Check sheet for the modelled part. Datum: model origin and axes. Units: mm. A direction names the side the tool comes from. Give positions to 0.01 mm unless a question says otherwise; leave off trailing zeros. Loops run counter-clockwise (first coordinate to the right, second up) from the corner with the lowest first, then second, coordinate; pieces in that order, holes last. Notation, with made-up numbers: (75, -10) -> (88, -10) arc R28 ccw to (88, 17) -> close; hole circle Ø2 at (-15, 65.25). An arc over 180 degrees is marked (long way). Answer as CSV lines item,"result". Start each with the question number.
(1) Material ranges on line 1 (X direction, y = -79, z = 9.25); line 2 (Y direction, x = -92, z = 9); line 3 (X direction, y = 85, z = 3.5), recorded low to high. Write a range as from..to.
(2) Section check A-A on x = 24. Enter the section's corners in (y, z).
(3) Section check B-B on y = 48. Enter the section's corners in (x, z).
(4) Access from +Z, -Z, +X, -X, +Y, -Y to the whole of each face (thin tool, end or side, straight path). Record for faces 1 (the face through (-130, -1, 12)), 2 (the face through (-2, -105, 0)), 3 (the face through (-2, -97, 8)), 4 (the face through (-2, 100, 12)), 5 (the face through (130, -1, 12)).
(5) Gauge pin test, flat ends, axial feed: pin 1 Ø5 at (x, z) = (33, 11) entering from -Y; pin 2 Ø8 at (y, z) = (-26, 9) entering from +X; pin 3 Ø4 at (y, z) = (-40.5, 12) entering from -X. Record the tip position at first contact, or that the pin passes through.
(6) Release check for a two-part mould opening along Y. For faces 6 (the face through (-2, -105, 4)), 7 (the face through (-2, -100, 12)), 8 (the face through (-2, 1, 16)) record: pulls with the +Y half, pulls with the -Y half, needs draft (parallel to the pull), parting line crosses it, or undercut.
from build123d import *

# Parameters (mm, degrees)
SKETCH1_W                = 300
SKETCH1_H                = 240
SKETCH1_W_2              = 260
SKETCH1_H_2              = 200
BOSS_EXTRUDE1_DEPTH      = 4
SKETCH2_W                = 260
SKETCH2_H                = 200
SKETCH2_W_2              = 252.2
SKETCH2_H_2              = 194
BOSS_EXTRUDE3_DEPTH      = 16
BOSS_EXTRUDE3_DEPTH_BACK = 4
SKETCH4_W                = 252.2
SKETCH4_H                = 194
BOSS_EXTRUDE4_DEPTH      = 4


with BuildPart() as part:
    # Sketch1 → Boss-Extrude1 (new body)
    with BuildSketch(Plane.XY):
        Rectangle(SKETCH1_W, SKETCH1_H)
        Rectangle(SKETCH1_W_2, SKETCH1_H_2, mode=Mode.SUBTRACT)
    extrude(amount=BOSS_EXTRUDE1_DEPTH)

    # Sketch2 → Boss-Extrude3 (add, two sides)
    with BuildSketch(Plane.XY.offset(4)) as boss_extrude3_sk:
        Rectangle(SKETCH2_W, SKETCH2_H)
        Rectangle(SKETCH2_W_2, SKETCH2_H_2, mode=Mode.SUBTRACT)
    extrude(amount=BOSS_EXTRUDE3_DEPTH)
    extrude(boss_extrude3_sk.sketch, amount=-BOSS_EXTRUDE3_DEPTH_BACK)

    # Sketch4 → Boss-Extrude4 (add)
    with BuildSketch(Plane.XY.offset(20)):
        Rectangle(SKETCH4_W, SKETCH4_H)
    extrude(amount=-BOSS_EXTRUDE4_DEPTH)


solid = part.part
Working result:
1,line 1,"x = -130..-126.1, 126.1..130"
1,line 2,"y = -100..-97, 97..100"
1,line 3,"x = -150..-126.1, 126.1..150"
2,outline,"(-120, 0) -> (-97, 0) -> (-97, 16) -> (97, 16) -> (97, 0) -> (120, 0) -> (120, 4) -> (100, 4) -> (100, 20) -> (-100, 20) -> (-100, 4) -> (-120, 4) -> close"
3,outline,"(-150, 0) -> (-126.1, 0) -> (-126.1, 16) -> (126.1, 16) -> (126.1, 0) -> (150, 0) -> (150, 4) -> (130, 4) -> (130, 20) -> (-130, 20) -> (-130, 4) -> (-150, 4) -> close"
4,face 1,"+Z, -X, +Y, -Y"
4,face 2,"-Z, +X, -X, +Y, -Y"
4,face 3,"-Z"
4,face 4,"+Z, +X, -X, +Y"
4,face 5,"+Z, +X, +Y, -Y"
5,pin 1,"stops at y = -100"
5,pin 2,"stops at x = 130"
5,pin 3,"stops at x = -130"
6,face 6,"needs draft"
6,face 7,"pulls with the -Y half"
6,face 8,"undercut"
